Work out the finished part from the listing and answer in its coordinate system (mm). Round coordinates to 2 decimals unless told otherwise and drop trailing zeros. Write each loop counter-clockwise with the first axis right and the second up, starting at its lowest first coordinate (ties: lowest second). Pieces come first, ordered by that corner, then holes.
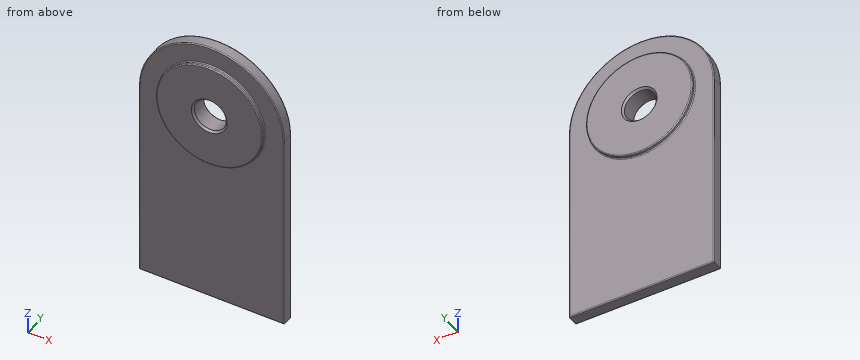
from build123d import *

# Parameters (mm, degrees)
F0_R     = 55
F1_DEPTH = 6
F0_R_2   = 16.5
F2_DEPTH = 10
F3_SIZE  = 2
F4_R     = 1
F5_R     = 1


with BuildPart() as f1:
    # F0 (on Front) → F1 (new body, symmetric)
    with BuildSketch(Plane.XZ):
        with BuildLine():
            Line((75, -210), (75, 0))
            ThreePointArc((75, 0), (0, 75), (-75, 0))
            Line((-75, 0), (-75, -210))
            Line((-75, -210), (75, -210))
        make_face()
        Circle(F0_R, mode=Mode.SUBTRACT)
    extrude(amount=F1_DEPTH, both=True)

    # F0 (on Front) → F2 (join, symmetric)
    with BuildSketch(Plane.XZ):
        Circle(F0_R)
        Circle(F0_R_2, mode=Mode.SUBTRACT)
    extrude(amount=F2_DEPTH, both=True)

    # F3
    f3_edges = [f1.edges().sort_by_distance(p)[0] for p in [
        (-16.5, -10, 0),
        (-16.5, 10, 0),
    ]]
    chamfer(f3_edges, length=F3_SIZE)

    # F4
    f4_edges = [f1.edges().sort_by_distance(p)[0] for p in [
        (-55, 10, 0),
        (-75, 6, -105),
        (0, 6, -210),
        (75, 6, -105),
        (0, 6, 75),
        (-55, 6, 0),
        (-75, -6, -105),
        (0, -6, -210),
        (75, -6, -105),
        (0, -6, 75),
        (-55, -6, 0),
    ]]
    fillet(f4_edges, radius=F4_R)

    # F5
    f5_edges = [f1.edges().sort_by_distance(p)[0] for p in [
        (-55, -10, 0),
    ]]
    fillet(f5_edges, radius=F5_R)


solid = f1.part
Q1. Given pin 1 (10 mm diameter, centred on x = -50.5, z = -68.5, fed in from +Y); pin 2 (6 mm diameter, centred on x = 10, z = -102, fed in from -Y); pin 3 (12 mm diameter, centred on x = 17, y = -2, fed in from +Z), each flat-ended and moving along its own axis, determine where each tip first touches the part or whether it passes through.
Q2. Find section C-C (y = 1.5). Determine the outline of the cut face in (x, z).
Q3. Find the intervals of material crossed by L1, parallel to Z at x = 0, y = 4.5; L2, parallel to Y at x = -26.5, z = -172; L3, parallel to X at y = 9, z = 0.5, in increasing order.
Q4. Find section B-B (z = -188). Determine the outline of the cut face in (x, y).
Report:
1. pin 1: stops at y = 6
1. pin 2: stops at y = -6
1. pin 3: stops at z = 74.19
2. outline: (-75, -210) - (75, -210) - (75, 0) arc R75 ccw to (-75, 0) - close; hole circle Ø33 at (0, 0)
3. L1: z = -210 to -16.5, 16.5 to 75
3. L2: y = -6 to 6
3. L3: x = -55 to -17.49, 17.49 to 55
4. outline: (-75, -5) arc R1 ccw to (-74, -6) - (74, -6) arc R1 ccw to (75, -5) - (75, 5) arc R1 ccw to (74, 6) - (-74, 6) arc R1 ccw to (-75, 5) - close
